For this review, take the finished solid that the model builds, in its own axes (mm). Coordinates: 2 decimals unless noted, no trailing zeros. Order: outer loops, then holes, each group sorted by start corner. A loop starts at its lowest first (then second) coordinate and runs counter-clockwise, first axis right, second up. Notation, with made-up numbers: (39, -12.5) - (43, -12.5) arc R30 ccw to (43, 11.5) - close; hole circle Ø1 at (-13.75, 56). An arc over 180 degrees is marked (long way). One line per item, written item: value. Start each with the question number.
(1) Consider section B-B on z = 0.7. Count the separate pieces of the cut face and the enclosed holes in it, then the cut area to 3 significant figures.
(2) Consider section A-A on x = 30. Write out the cut boundary in (y, z), then the cut area to 3 significant figures.
(3) To check wall thickness, follow line 1 along X through (y, z) = (22, 1.6); line 2 along Y through (x, z) = (-19, 0.85); line 3 along Y through (x, z) = (-57.5, 2.35). State the ranges of each line that lie inside material, in increasing order.
(4) Clearance check with flat-ended pins moving along their axes: pin 1 (3 mm diameter, centred on x = 0, y = -45, fed in from -Z); pin 2 (2.5 mm diameter, centred on x = 19, y = -15, fed in from +Z) (3 decimals). State where each tip first meets the part, or that it passes through.
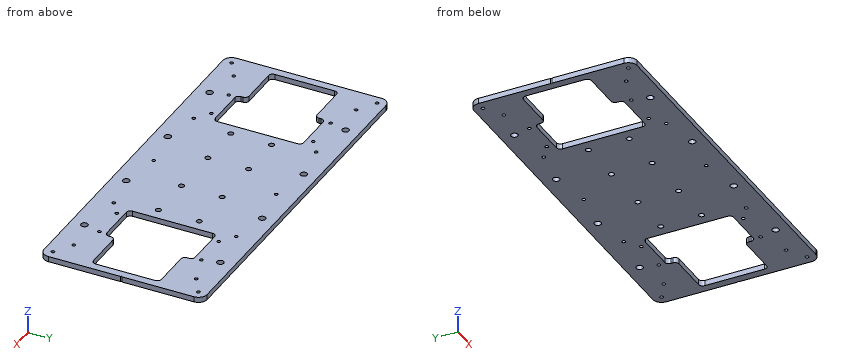
```python
from build123d import *

# Parameters (mm, degrees)
ESQUISSE1_W             = 135
ESQUISSE1_H             = 120
BOSS_EXTRU_1_DEPTH      = 4
ENL_V_MAT_EXTRU_1_REACH = 149.787
CONG_1_R                = 3
ENL_V_MAT_EXTRU_2_REACH = 149.787
ESQUISSE3_R             = 2.5
ESQUISSE3_R_2           = 1.25
ESQUISSE3_R_3           = 0.5
ESQUISSE3_R_4           = 2
ENL_V_MAT_EXTRU_3_REACH = 149.787
ESQUISSE4_R             = 1.25
CONG_2_R                = 6.5


with BuildPart() as part:
    # Esquisse1 → Boss.-Extru.1 (new body)
    with BuildSketch(Plane.XY):
        with Locations((67.5, 0)):
            Rectangle(ESQUISSE1_W, ESQUISSE1_H)
    extrude(amount=BOSS_EXTRU_1_DEPTH)

    # Esquisse2 → Enlèv. mat.-Extru.1 (cut, up to next)
    with BuildSketch(Plane.XY.offset(4), mode=Mode.PRIVATE) as enl_v_mat_extru_1_sk1:
        Polygon((95, -25), (95, -32.5), (61, -32.5), (61, 32.5), (95, 32.5), (95, 25), (129, 25), (129, -25), align=None)
    enl_v_mat_extru_1_tool1 = extrude(enl_v_mat_extru_1_sk1.sketch, amount=-ENL_V_MAT_EXTRU_1_REACH, mode=Mode.PRIVATE) & part.part
    add(enl_v_mat_extru_1_tool1.solids().sort_by_distance((92.782609, 0, 4))[0], mode=Mode.SUBTRACT)

    # Congé1
    cong_1_edges = [part.edges().sort_by_distance(p)[0] for p in [
        (95, 32.5, 2),
        (95, 25, 2),
        (129, 25, 2),
        (129, -25, 2),
        (95, -25, 2),
        (95, -32.5, 2),
        (61, -32.5, 2),
        (61, 32.5, 2),
    ]]
    fillet(cong_1_edges, radius=CONG_1_R)

    # Esquisse3 → Enlèv. mat.-Extru.2 (cut, up to next)
    with BuildSketch(Plane.XY.offset(4), mode=Mode.PRIVATE) as enl_v_mat_extru_2_sk1:
        with Locations((30, 50)):
            Circle(ESQUISSE3_R)
    enl_v_mat_extru_2_tool1 = extrude(enl_v_mat_extru_2_sk1.sketch, amount=-ENL_V_MAT_EXTRU_2_REACH, mode=Mode.PRIVATE) & part.part
    # Esquisse3 → Enlèv. mat.-Extru.2 (cut, up to next)
    with BuildSketch(Plane.XY.offset(4), mode=Mode.PRIVATE) as enl_v_mat_extru_2_sk2:
        with Locations((90, 50)):
            Circle(ESQUISSE3_R)
    enl_v_mat_extru_2_tool2 = extrude(enl_v_mat_extru_2_sk2.sketch, amount=-ENL_V_MAT_EXTRU_2_REACH, mode=Mode.PRIVATE) & part.part
    # Esquisse3 → Enlèv. mat.-Extru.2 (cut, up to next)
    with BuildSketch(Plane.XY.offset(4), mode=Mode.PRIVATE) as enl_v_mat_extru_2_sk3:
        with Locations((90, -50)):
            Circle(ESQUISSE3_R)
    enl_v_mat_extru_2_tool3 = extrude(enl_v_mat_extru_2_sk3.sketch, amount=-ENL_V_MAT_EXTRU_2_REACH, mode=Mode.PRIVATE) & part.part
    # Esquisse3 → Enlèv. mat.-Extru.2 (cut, up to next)
    with BuildSketch(Plane.XY.offset(4), mode=Mode.PRIVATE) as enl_v_mat_extru_2_sk4:
        with Locations((30, -50)):
            Circle(ESQUISSE3_R)
    enl_v_mat_extru_2_tool4 = extrude(enl_v_mat_extru_2_sk4.sketch, amount=-ENL_V_MAT_EXTRU_2_REACH, mode=Mode.PRIVATE) & part.part
    # Esquisse3 → Enlèv. mat.-Extru.2 (cut, up to next)
    with BuildSketch(Plane.XY.offset(4), mode=Mode.PRIVATE) as enl_v_mat_extru_2_sk5:
        with Locations((0, 45)):
            Circle(ESQUISSE3_R_2)
    enl_v_mat_extru_2_tool5 = extrude(enl_v_mat_extru_2_sk5.sketch, amount=-ENL_V_MAT_EXTRU_2_REACH, mode=Mode.PRIVATE) & part.part
    # Esquisse3 → Enlèv. mat.-Extru.2 (cut, up to next)
    with BuildSketch(Plane.XY.offset(4), mode=Mode.PRIVATE) as enl_v_mat_extru_2_sk6:
        with Locations((115, 45)):
            Circle(ESQUISSE3_R_2)
    enl_v_mat_extru_2_tool6 = extrude(enl_v_mat_extru_2_sk6.sketch, amount=-ENL_V_MAT_EXTRU_2_REACH, mode=Mode.PRIVATE) & part.part
    # Esquisse3 → Enlèv. mat.-Extru.2 (cut, up to next)
    with BuildSketch(Plane.XY.offset(4), mode=Mode.PRIVATE) as enl_v_mat_extru_2_sk7:
        with Locations((115, -45)):
            Circle(ESQUISSE3_R_2)
    enl_v_mat_extru_2_tool7 = extrude(enl_v_mat_extru_2_sk7.sketch, amount=-ENL_V_MAT_EXTRU_2_REACH, mode=Mode.PRIVATE) & part.part
    # Esquisse3 → Enlèv. mat.-Extru.2 (cut, up to next)
    with BuildSketch(Plane.XY.offset(4), mode=Mode.PRIVATE) as enl_v_mat_extru_2_sk8:
        with Locations((0, -45)):
            Circle(ESQUISSE3_R_2)
    enl_v_mat_extru_2_tool8 = extrude(enl_v_mat_extru_2_sk8.sketch, amount=-ENL_V_MAT_EXTRU_2_REACH, mode=Mode.PRIVATE) & part.part
    # Esquisse3 → Enlèv. mat.-Extru.2 (cut, up to next)
    with BuildSketch(Plane.XY.offset(4), mode=Mode.PRIVATE) as enl_v_mat_extru_2_sk9:
        with Locations((57.5, -45)):
            Circle(ESQUISSE3_R_2)
    enl_v_mat_extru_2_tool9 = extrude(enl_v_mat_extru_2_sk9.sketch, amount=-ENL_V_MAT_EXTRU_2_REACH, mode=Mode.PRIVATE) & part.part
    # Esquisse3 → Enlèv. mat.-Extru.2 (cut, up to next)
    with BuildSketch(Plane.XY.offset(4), mode=Mode.PRIVATE) as enl_v_mat_extru_2_sk10:
        with Locations((57.5, 45)):
            Circle(ESQUISSE3_R_2)
    enl_v_mat_extru_2_tool10 = extrude(enl_v_mat_extru_2_sk10.sketch, amount=-ENL_V_MAT_EXTRU_2_REACH, mode=Mode.PRIVATE) & part.part
    # Esquisse3 → Enlèv. mat.-Extru.2 (cut, up to next)
    with BuildSketch(Plane.XY.offset(4), mode=Mode.PRIVATE) as enl_v_mat_extru_2_sk11:
        with Locations((128.5, 53.5)):
            Circle(ESQUISSE3_R_2)
    enl_v_mat_extru_2_tool11 = extrude(enl_v_mat_extru_2_sk11.sketch, amount=-ENL_V_MAT_EXTRU_2_REACH, mode=Mode.PRIVATE) & part.part
    # Esquisse3 → Enlèv. mat.-Extru.2 (cut, up to next)
    with BuildSketch(Plane.XY.offset(4), mode=Mode.PRIVATE) as enl_v_mat_extru_2_sk12:
        with Locations((128.5, -53.5)):
            Circle(ESQUISSE3_R_2)
    enl_v_mat_extru_2_tool12 = extrude(enl_v_mat_extru_2_sk12.sketch, amount=-ENL_V_MAT_EXTRU_2_REACH, mode=Mode.PRIVATE) & part.part
    # Esquisse3 → Enlèv. mat.-Extru.2 (cut, up to next)
    with BuildSketch(Plane.XY.offset(4), mode=Mode.PRIVATE) as enl_v_mat_extru_2_sk13:
        with Locations((135, 0)):
            Circle(ESQUISSE3_R_3)
    enl_v_mat_extru_2_tool13 = extrude(enl_v_mat_extru_2_sk13.sketch, amount=-ENL_V_MAT_EXTRU_2_REACH, mode=Mode.PRIVATE) & part.part
    # Esquisse3 → Enlèv. mat.-Extru.2 (cut, up to next)
    with BuildSketch(Plane.XY.offset(4), mode=Mode.PRIVATE) as enl_v_mat_extru_2_sk14:
        with Locations((52, 15)):
            Circle(ESQUISSE3_R_4)
    enl_v_mat_extru_2_tool14 = extrude(enl_v_mat_extru_2_sk14.sketch, amount=-ENL_V_MAT_EXTRU_2_REACH, mode=Mode.PRIVATE) & part.part
    # Esquisse3 → Enlèv. mat.-Extru.2 (cut, up to next)
    with BuildSketch(Plane.XY.offset(4), mode=Mode.PRIVATE) as enl_v_mat_extru_2_sk15:
        with Locations((19, 15)):
            Circle(ESQUISSE3_R_4)
    enl_v_mat_extru_2_tool15 = extrude(enl_v_mat_extru_2_sk15.sketch, amount=-ENL_V_MAT_EXTRU_2_REACH, mode=Mode.PRIVATE) & part.part
    # Esquisse3 → Enlèv. mat.-Extru.2 (cut, up to next)
    with BuildSketch(Plane.XY.offset(4), mode=Mode.PRIVATE) as enl_v_mat_extru_2_sk16:
        with Locations((19, -15)):
            Circle(ESQUISSE3_R_4)
    enl_v_mat_extru_2_tool16 = extrude(enl_v_mat_extru_2_sk16.sketch, amount=-ENL_V_MAT_EXTRU_2_REACH, mode=Mode.PRIVATE) & part.part
    # Esquisse3 → Enlèv. mat.-Extru.2 (cut, up to next)
    with BuildSketch(Plane.XY.offset(4), mode=Mode.PRIVATE) as enl_v_mat_extru_2_sk17:
        with Locations((52, -15)):
            Circle(ESQUISSE3_R_4)
    enl_v_mat_extru_2_tool17 = extrude(enl_v_mat_extru_2_sk17.sketch, amount=-ENL_V_MAT_EXTRU_2_REACH, mode=Mode.PRIVATE) & part.part
    add(enl_v_mat_extru_2_tool1.solids().sort_by_distance((30, 50, 4))[0], mode=Mode.SUBTRACT)
    add(enl_v_mat_extru_2_tool2.solids().sort_by_distance((90, 50, 4))[0], mode=Mode.SUBTRACT)
    add(enl_v_mat_extru_2_tool3.solids().sort_by_distance((90, -50, 4))[0], mode=Mode.SUBTRACT)
    add(enl_v_mat_extru_2_tool4.solids().sort_by_distance((30, -50, 4))[0], mode=Mode.SUBTRACT)
    add(enl_v_mat_extru_2_tool5.solids().sort_by_distance((0, 45, 4))[0], mode=Mode.SUBTRACT)
    add(enl_v_mat_extru_2_tool6.solids().sort_by_distance((115, 45, 4))[0], mode=Mode.SUBTRACT)
    add(enl_v_mat_extru_2_tool7.solids().sort_by_distance((115, -45, 4))[0], mode=Mode.SUBTRACT)
    add(enl_v_mat_extru_2_tool8.solids().sort_by_distance((0, -45, 4))[0], mode=Mode.SUBTRACT)
    add(enl_v_mat_extru_2_tool9.solids().sort_by_distance((57.5, -45, 4))[0], mode=Mode.SUBTRACT)
    add(enl_v_mat_extru_2_tool10.solids().sort_by_distance((57.5, 45, 4))[0], mode=Mode.SUBTRACT)
    add(enl_v_mat_extru_2_tool11.solids().sort_by_distance((128.5, 53.5, 4))[0], mode=Mode.SUBTRACT)
    add(enl_v_mat_extru_2_tool12.solids().sort_by_distance((128.5, -53.5, 4))[0], mode=Mode.SUBTRACT)
    add(enl_v_mat_extru_2_tool13.solids().sort_by_distance((135, 0, 4))[0], mode=Mode.SUBTRACT)
    add(enl_v_mat_extru_2_tool14.solids().sort_by_distance((52, 15, 4))[0], mode=Mode.SUBTRACT)
    add(enl_v_mat_extru_2_tool15.solids().sort_by_distance((19, 15, 4))[0], mode=Mode.SUBTRACT)
    add(enl_v_mat_extru_2_tool16.solids().sort_by_distance((19, -15, 4))[0], mode=Mode.SUBTRACT)
    add(enl_v_mat_extru_2_tool17.solids().sort_by_distance((52, -15, 4))[0], mode=Mode.SUBTRACT)

    # Esquisse4 → Enlèv. mat.-Extru.3 (cut, up to next)
    with BuildSketch(Plane.XY.offset(4), mode=Mode.PRIVATE) as enl_v_mat_extru_3_sk1:
        with Locations((68, 37.5)):
            Circle(ESQUISSE4_R)
    enl_v_mat_extru_3_tool1 = extrude(enl_v_mat_extru_3_sk1.sketch, amount=-ENL_V_MAT_EXTRU_3_REACH, mode=Mode.PRIVATE) & part.part
    # Esquisse4 → Enlèv. mat.-Extru.3 (cut, up to next)
    with BuildSketch(Plane.XY.offset(4), mode=Mode.PRIVATE) as enl_v_mat_extru_3_sk2:
        with Locations((93, 37.5)):
            Circle(ESQUISSE4_R)
    enl_v_mat_extru_3_tool2 = extrude(enl_v_mat_extru_3_sk2.sketch, amount=-ENL_V_MAT_EXTRU_3_REACH, mode=Mode.PRIVATE) & part.part
    # Esquisse4 → Enlèv. mat.-Extru.3 (cut, up to next)
    with BuildSketch(Plane.XY.offset(4), mode=Mode.PRIVATE) as enl_v_mat_extru_3_sk3:
        with Locations((68, -37.5)):
            Circle(ESQUISSE4_R)
    enl_v_mat_extru_3_tool3 = extrude(enl_v_mat_extru_3_sk3.sketch, amount=-ENL_V_MAT_EXTRU_3_REACH, mode=Mode.PRIVATE) & part.part
    # Esquisse4 → Enlèv. mat.-Extru.3 (cut, up to next)
    with BuildSketch(Plane.XY.offset(4), mode=Mode.PRIVATE) as enl_v_mat_extru_3_sk4:
        with Locations((93, -37.5)):
            Circle(ESQUISSE4_R)
    enl_v_mat_extru_3_tool4 = extrude(enl_v_mat_extru_3_sk4.sketch, amount=-ENL_V_MAT_EXTRU_3_REACH, mode=Mode.PRIVATE) & part.part
    add(enl_v_mat_extru_3_tool1.solids().sort_by_distance((68, 37.5, 4))[0], mode=Mode.SUBTRACT)
    add(enl_v_mat_extru_3_tool2.solids().sort_by_distance((93, 37.5, 4))[0], mode=Mode.SUBTRACT)
    add(enl_v_mat_extru_3_tool3.solids().sort_by_distance((68, -37.5, 4))[0], mode=Mode.SUBTRACT)
    add(enl_v_mat_extru_3_tool4.solids().sort_by_distance((93, -37.5, 4))[0], mode=Mode.SUBTRACT)

    # Congé2
    cong_2_edges = [part.edges().sort_by_distance(p)[0] for p in [
        (135, -60, 2),
        (135, 60, 2),
    ]]
    fillet(cong_2_edges, radius=CONG_2_R)

    # Symétrie1: part across plane


with BuildPart() as part_1:
    add(part.part)
    add(part.part.mirror(Plane(origin=(0, 60, 4), x_dir=(0, 0, 1), z_dir=(1, 0, 0))))


solid = part_1.part
```
Geometry check:
1. separate pieces: 1
1. enclosed holes: 40
1. area: 24,200 mm^2
2. outline: (-60, 0) - (-52.5, 0) - (-52.5, 4) - (-60, 4) - close; (-47.5, 0) - (47.5, 0) - (47.5, 4) - (-47.5, 4) - close; (52.5, 0) - (60, 0) - (60, 4) - (52.5, 4) - close
2. area: 440 mm^2
3. line 1: x = -135 to -129, -61 to 61, 129 to 135
3. line 2: y = -60 to -17, -13 to 13, 17 to 60
3. line 3: y = -60 to -46.25, -43.75 to 43.75, 46.25 to 60
4. pin 1: stops at z = 0
4. pin 2: passes through
